from build123d import *

# Parameters (mm, degrees)
SKETCH1_R           = 62.5
BOSS_EXTRUDE1_DEPTH = 60
SKETCH2_R           = 57.5
CUT_EXTRUDE1_DEPTH  = 56
SKETCH3_R           = 12.7
BOSS_EXTRUDE2_DEPTH = 13.11
SKETCH4_R           = 1.75
SKETCH4_R_2         = 3
CUT_EXTRUDE2_DEPTH  = 99.244857881
SKETCH5_R           = 3.25
CUT_EXTRUDE3_DEPTH  = 3
FILLET1_R           = 5
FILLET2_R           = 10


with BuildPart() as part:
    # Sketch1 → Boss-Extrude1 (new body)
    with BuildSketch(Plane.XY):
        Circle(SKETCH1_R)
    extrude(amount=BOSS_EXTRUDE1_DEPTH)

    # Sketch2 → Cut-Extrude1 (cut)
    with BuildSketch(Plane.XY.offset(60)):
        Circle(SKETCH2_R)
    extrude(amount=-CUT_EXTRUDE1_DEPTH, mode=Mode.SUBTRACT)

    # Sketch3 → Boss-Extrude2 (add)
    with BuildSketch(Plane.XY.offset(4)):
        Circle(SKETCH3_R)
    extrude(amount=BOSS_EXTRUDE2_DEPTH)

    # Sketch4 → Cut-Extrude2 (cut, through all)
    with BuildSketch(Plane.XY.offset(17.11)):
        with Locations((-5.784301124, 7.536037454)):
            Circle(SKETCH4_R)
        with Locations((-9.418550441, -1.24133299)):
            Circle(SKETCH4_R)
        with Locations((-3.634249317, -8.777370444)):
            Circle(SKETCH4_R)
        with Locations((5.784301124, -7.536037454)):
            Circle(SKETCH4_R)
        with Locations((9.418550441, 1.24133299)):
            Circle(SKETCH4_R)
        with Locations((3.634249317, 8.777370444)):
            Circle(SKETCH4_R)
        Circle(SKETCH4_R_2)
    extrude(amount=-CUT_EXTRUDE2_DEPTH, mode=Mode.SUBTRACT)

    # Sketch5 → Cut-Extrude3 (cut)
    with BuildSketch(Plane(origin=(0, 0, 0), x_dir=(-1, 0, 0), z_dir=(0, 0, -1))):
        with Locations((-9.418550441, 1.24133299)):
            Circle(SKETCH5_R)
        with Locations((-3.634249317, 8.777370444)):
            Circle(SKETCH5_R)
        with Locations((5.784301124, 7.536037454)):
            Circle(SKETCH5_R)
        with Locations((9.418550441, -1.24133299)):
            Circle(SKETCH5_R)
        with Locations((3.634249317, -8.777370444)):
            Circle(SKETCH5_R)
        with Locations((-5.784301124, -7.536037454)):
            Circle(SKETCH5_R)
    extrude(amount=-CUT_EXTRUDE3_DEPTH, mode=Mode.SUBTRACT)

    # Fillet1
    fillet1_edges = [part.edges().sort_by_distance(p)[0] for p in [
        (-57.5, 0, 4),
    ]]
    fillet(fillet1_edges, radius=FILLET1_R)

    # Fillet2
    fillet2_edges = [part.edges().sort_by_distance(p)[0] for p in [
        (-12.7, 0, 4),
    ]]
    fillet(fillet2_edges, radius=FILLET2_R)


solid = part.part
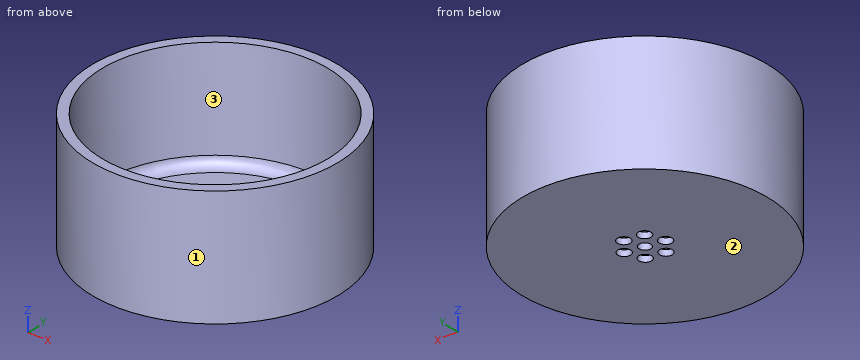
Work out the finished part from the listing and answer in its coordinate system (mm). Face numbers are marked on the shaded views. Coordinates: 2 decimals unless noted, no trailing zeros. Loops run counter-clockwise (first coordinate to the right, second up) from the corner with the lowest first, then second, coordinate; pieces in that order, holes last. Notation, with made-up numbers: (55, 35.5) -> (113, 35.5) arc R20 cw to (113, 56.5) -> close; hole circle Ø10 at (65, 55). An arc over 180 degrees is marked (long way). Write each question's results on one line, items separated by ' | '. Start each with the question number.
1) The mould has two halves that part along Y. Classify the marked faces 1, 2 and 3: pulls with the +Y half, pulls with the -Y half, needs draft (parallel to the pull), parting line crosses it, or undercut.
2) Find section A-A on z = 41. Determine the outline of the cut face in (x, y).
3) Flat-ended cylindrical pins translate along their axes: P1, Ø3, axis at y = 43.5, z = 36, coming from the +X side; P2, Ø1.5, axis at y = -10, z = 26.5, coming from the +X side; P3, Ø5, axis at x = -14, y = -21.5, coming from the +Z side. Find the tip coordinate at first contact, or state that the pin passes through.
4) Consider line 1 along Y through (x, z) = (0, 45); line 2 along Y through (x, z) = (0, 9); line 3 along Z through (x, y) = (25, -8). Determine where each line is inside the solid, lowest interval first.
Response values:
1) face 1: parting line crosses it | face 2: needs draft | face 3: undercut
2) outline: circle Ø125 at (0, 0); hole circle Ø115 at (0, 0)
3) P1: stops at x = 46.28 | P2: stops at x = 61.81 | P3: stops at z = 4
4) line 1: y = -62.5 to -57.5, 57.5 to 62.5 | line 2: y = -62.5 to -57.5, -14.04 to -3, 3 to 14.04, 57.5 to 62.5 | line 3: z = 0 to 4
